Can you work these out from the drawing? Everything is in mm from the part's minimum corner. A direction names the side the tool comes from. Coordinates: 2 decimals unless noted, no trailing zeros. Order: outer loops, then holes, each group sorted by start corner. A loop starts at its lowest first (then second) coordinate and runs counter-clockwise, first axis right, second up. Notation, with made-up numbers: (1.25, 55.5) -> (6.25, 55.5) arc R10 ccw to (6.25, 59.5) -> close; hole circle Ø11 at (61, 58.5). An arc over 180 degrees is marked (long way). Use a Markdown table: item, result. Add a question column.
1) If I drill on L1, parallel to Z at x = 145, y = 73.5; L2, parallel to Y at x = 153, z = 129; L3, parallel to X at y = 33, z = 20, over which ranges is the centre line in solid material (lowest first)? Write a range as [from, to].
2) If we section it at D-D (y = 28.5): Write out the boundary of the cut face in (x, z).
3) If we section it at A-A (x = 145): Write out the boundary of the cut face in (y, z), plus the area to 3 significant figures.
4) If we section it at B-B (z = 69.5): Write out the boundary of the cut face in (x, y), plus the area to 3 significant figures.
5) Will these pins go through, and if not, where does the flat tip stop? pin 1 Ø1 at (x, z) = (103, 126) entering from -Y; pin 2 Ø10.5 at (x, y) = (52, 19) entering from +Z; pin 3 Ø24 at (x, z) = (145, 20) entering from +Y; pin 4 Ø1.5 at (y, z) = (26.5, 108.5) entering from -X.
6) Thinking about a two-plate mould opening in X: for the marked faces 1, 2 and 3, which applies, +X half, -X half, draft (parallel to the pull), parting line (faces both ways), or undercut?
7) If we section it at C-C (x = 117): Write out the boundary of the cut face in (y, z).
8) Which directions (+Z, -Z, +X, -X, +Y, -Y) give clear straight access to the entire face, cutting with the end or side of a thin tool? Please do the marked faces 4 and 5.
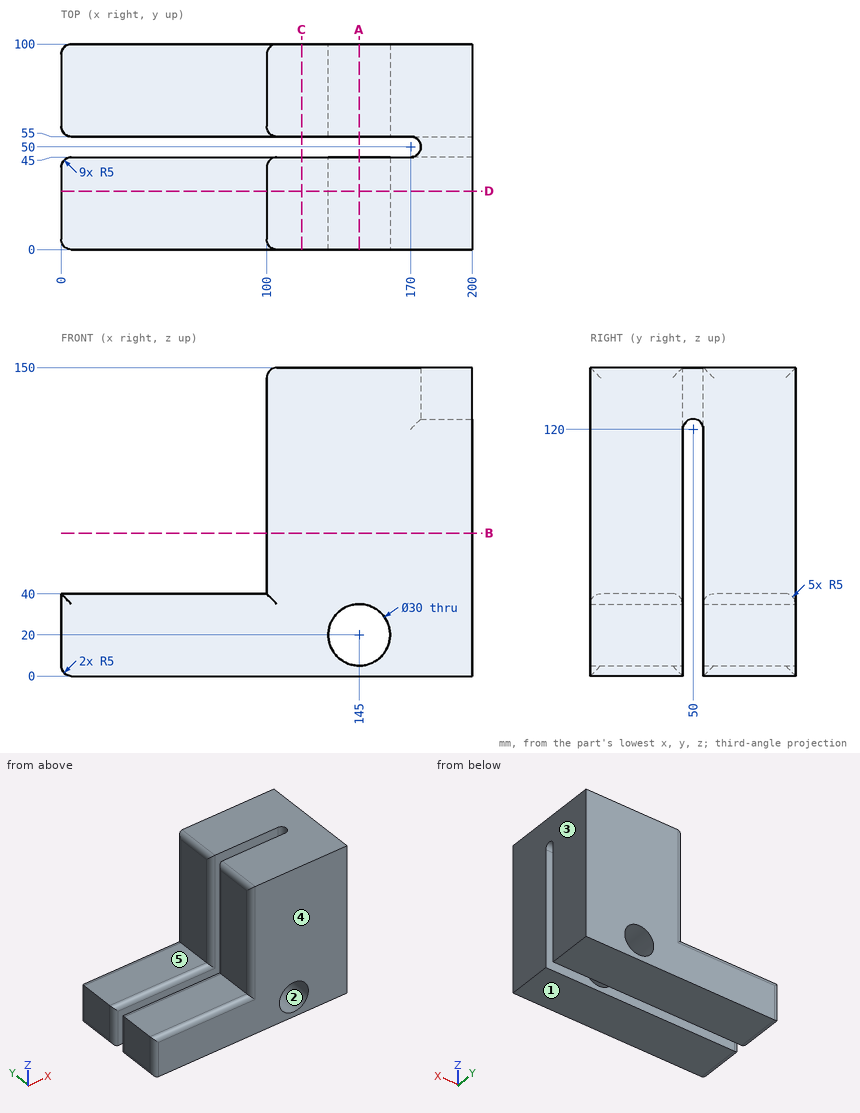
Answer sheet:
| question | item | result |
|---|---|---|
| 1 | L1 | [0, 5], [35, 150] |
| 1 | L2 | [0, 45], [55, 100] |
| 1 | L3 | [0, 130], [160, 200] |
| 2 | outline | (0, 5) arc R5 ccw to (5, 0) -> (200, 0) -> (200, 150) -> (105, 150) arc R5 ccw to (100, 145) -> (100, 40) -> (0, 40) -> close; hole circle Ø30 at (145, 20) |
| 3 | outline | (0, 0) -> (45, 0) -> (45, 5) -> (0, 5) -> close; (0, 35) -> (45, 35) -> (45, 150) -> (0, 150) -> close; (55, 0) -> (100, 0) -> (100, 5) -> (55, 5) -> close; (55, 35) -> (100, 35) -> (100, 150) -> (55, 150) -> close |
| 3 | area | 10,800 mm2 |
| 4 | outline | (100, 5) arc R5 ccw to (105, 0) -> (200, 0) -> (200, 45) -> (105, 45) arc R5 ccw to (100, 40) -> close; (100, 60) arc R5 ccw to (105, 55) -> (200, 55) -> (200, 100) -> (105, 100) arc R5 ccw to (100, 95) -> close |
| 4 | area | 8,980 mm2 |
| 5 | pin 1 | y = 0.23 |
| 5 | pin 2 | z = 40 |
| 5 | pin 3 | through |
| 5 | pin 4 | x = 100 |
| 6 | face 1 | draft |
| 6 | face 2 | undercut |
| 6 | face 3 | +X half |
| 7 | outline | (0, 0) -> (45, 0) -> (45, 150) -> (0, 150) -> close; (55, 0) -> (100, 0) -> (100, 150) -> (55, 150) -> close |
| 8 | face 4 | +Z, -Z, +X, -X, -Y |
| 8 | face 5 | +Z, -X, +Y, -Y |
